Source: CAD feature listing. Evaluate the final solid. Frame: model axes, mm. Face numbers are marked on the shaded views. Round coordinates to 2 decimals unless told otherwise and drop trailing zeros. Order: outer loops, then holes, each group sorted by start corner. A loop starts at its lowest first (then second) coordinate and runs counter-clockwise, first axis right, second up. Notation, with made-up numbers: (49, -35.5) -> (56, -35.5) arc R20 cw to (56, -7.5) -> close; hole circle Ø1 at (35.5, 61.5). An arc over 180 degrees is marked (long way). Use a Markdown table: item, result. Add a question column.
Autodesk Inventor part; units mm, degrees
ref_plane "YZ Plane" through (0, 0, 0) normal (1, 0, 0) x (0, 1, 0)
ref_plane "XZ Plane" through (0, 0, 0) normal (0, 1, 0) x (-1, 0, 0)
ref_plane "XY Plane" through (0, 0, 0) normal (0, 0, 1) x (1, 0, 0)
sketch "Sketch1" plane through (0, 0, 0) normal (0, 1, 0) x (-1, 0, 0)
  circle A0 centre (0, 0) radius 1
  circle A1 centre (0, 4) radius 0.7
  circle A2 centre (0, -10) radius 1.7
  circle A3 centre (0, 8) radius 0.5
  circle A4 centre (0, -5) radius 1.25
  line L0 (5, 12) -> (-5, 12)
  line L1 (-5, 12) -> (-5, -15)
  line L2 (-5, -15) -> (5, -15)
  line L3 (5, -15) -> (5, 12)
  dimension "d0" = 2
  dimension "d1" = 1.4
  dimension "d2" = 3.4
  dimension "d3" = 1
  dimension "d4" = 2.5
  dimension "d5" = 4
  dimension "d6" = 4
  dimension "d7" = 5
  dimension "d8" = 5
  dimension "d11" = 4
  dimension "d12" = 5
  dimension "d13" = 5
  dimension "d14" = 5
extrude "Extrusion1" add sketch "Sketch1" along normal blind 4
fillet "Fillet1" radius 3 4 edges at (5, 2, 12) (-5, 2, 12) (-5, 2, -15) (5, 2, -15)
chamfer "Chamfer1" distance 0.5 angle 45 5 edges at (1.7, 4, -10) (1.25, 4, -5) (1, 4, 0) (0.7, 4, 4) (0.5, 4, 8)
properties part number "hole_size_test"
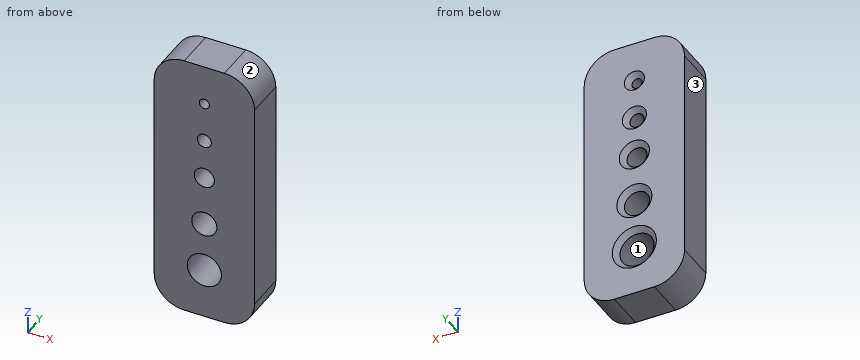
1) Section C-C on y = 1.2. Output: boundary loops of the cut face in (x, z), then the cut area to 3 significant figures.
2) Section A-A on z = 0. Output: boundary loops of the cut face in (x, y).
3) Line query: probe 1 along Z at (x, y) = (0, 0.95); probe 2 along X at (y, z) = (1.6, -5.25); probe 3 along X at (y, z) = (0.75, 0.5). Output: solid intervals per line, ascending. Write a range as from..to.
4) First-contact query: pin 1 Ø1.1 at (x, z) = (0, 4) entering from -Y; pin 2 Ø2.5 at (x, z) = (0, 0) entering from +Y. Flat tips, straight axial feed; report the tip coordinate or a pass-through.
5) Section D-D on z = -10. Output: boundary loops of the cut face in (x, y), then the cut area to 4 significant figures.
6) Draft query along X for the marked faces 1, 2 and 3. Return one class per face: pulls with the +X half, pulls with the -X half, needs draft (parallel to the pull), parting line crosses it, or undercut.
7) Section B-B on x = 0. Count the separate pieces of the cut face and the enclosed holes in it, then the cut area to 4 significant figures.
Conclusion:
| question | item | result |
|---|---|---|
| 1 | outline | (-5, -12) arc R3 ccw to (-2, -15) -> (2, -15) arc R3 ccw to (5, -12) -> (5, 9) arc R3 ccw to (2, 12) -> (-2, 12) arc R3 ccw to (-5, 9) -> close; hole circle Ø3.4 at (0, -10); hole circle Ø2.5 at (0, -5); hole circle Ø2 at (0, 0); hole circle Ø1.4 at (0, 4); hole circle Ø1 at (0, 8) |
| 1 | area | 243 mm^2 |
| 2 | outline | (-5, 0) -> (-1, 0) -> (-1, 3.5) -> (-1.5, 4) -> (-5, 4) -> close; (1, 0) -> (5, 0) -> (5, 4) -> (1.5, 4) -> (1, 3.5) -> close |
| 3 | probe 1 | z = -15..-11.7, -8.3..-6.25, -3.75..-1, 1..3.3, 4.7..7.5, 8.5..12 |
| 3 | probe 2 | x = -5..-1.22, 1.22..5 |
| 3 | probe 3 | x = -5..-0.87, 0.87..5 |
| 4 | pin 1 | passes through |
| 4 | pin 2 | stops at y = 3.75 |
| 5 | outline | (-5, 0) -> (-1.7, 0) -> (-1.7, 3.5) -> (-2.2, 4) -> (-5, 4) -> close; (1.7, 0) -> (5, 0) -> (5, 4) -> (2.2, 4) -> (1.7, 3.5) -> close |
| 5 | area | 26.15 mm^2 |
| 6 | face 1 | undercut |
| 6 | face 2 | pulls with the +X half |
| 6 | face 3 | pulls with the -X half |
| 7 | separate pieces | 6 |
| 7 | enclosed holes | 0 |
| 7 | area | 65.55 mm^2 |
